Can you work these out from the drawing? Everything is in mm from the part's minimum corner. A direction names the side the tool comes from. Round coordinates to 2 decimals unless told otherwise and drop trailing zeros. Order: outer loops, then holes, each group sorted by start corner. A loop starts at its lowest first (then second) coordinate and runs counter-clockwise, first axis right, second up. Notation, with made-up numbers: (49, -14.75) -> (78, -14.75) arc R23 ccw to (78, 1.25) -> close; hole circle Ø4 at (-34.75, -30). An arc over 180 degrees is marked (long way). One line per item, written item: value.
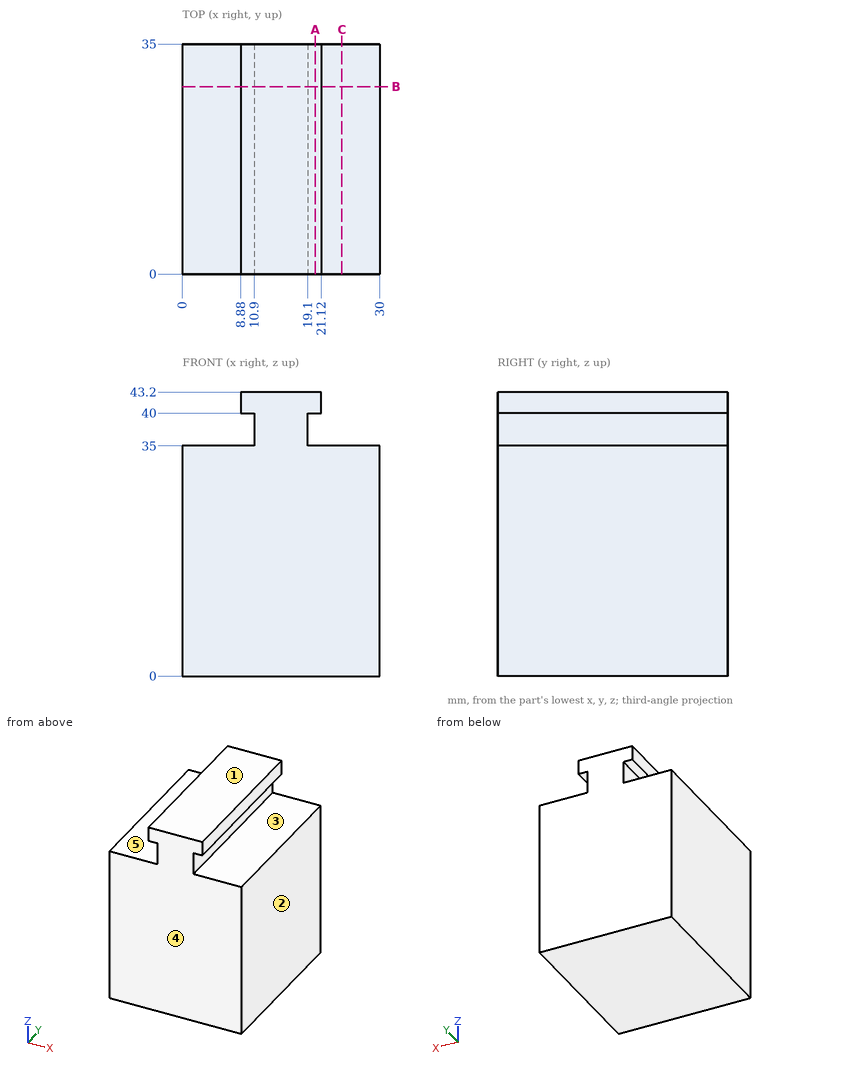
Q1. Which directions (+Z, -Z, +X, -X, +Y, -Y) give clear straight access to the entire face, cutting with the end or side of a thin tool? Please do the marked faces 4 and 5.
Answers:
face 4: +Z, -Z, +X, -X, -Y
face 5: -X, +Y, -Y
Q2. I want a section at C-C on x = 24.25. Write out the boundary of the cut face in (y, z), then the cut area to 4 significant figures.
Answers:
outline: (0, 0) -> (35, 0) -> (35, 35) -> (0, 35) -> close
area: 1,225 mm2
Q3. For P1, Ø2.5, axis at y = 22, z = 38, coming from the +X side; P2, Ø5.5, axis at y = 18, z = 38.5, coming from the -X side; P3, Ø1, axis at x = 22.5, y = 9, coming from the +Z side, each with a flat end and sliding along its axis, tell me the tip position at first contact or that it passes through.
Answers:
P1: x = 19.1
P2: x = 8.88
P3: z = 35
Q4. I want a section at B-B on y = 28.5. Write out the boundary of the cut face in (x, z).
Answers:
outline: (0, 0) -> (30, 0) -> (30, 35) -> (19.1, 35) -> (19.1, 40) -> (21.12, 40) -> (21.12, 43.2) -> (8.88, 43.2) -> (8.88, 40) -> (10.9, 40) -> (10.9, 35) -> (0, 35) -> close
Q5. If we mould it in two halves opening along Z, with no side actions, what happens to the marked faces 1, 2 and 3? For each: pulls with the +Z half, pulls with the -Z half, needs draft (parallel to the pull), parting line crosses it, or undercut.
Answers:
face 1: pulls with the +Z half
face 2: needs draft
face 3: undercut
Q6. I need wall thicknesses on line 1 along Z through (x, y) = (3, 16.5); line 2 along X through (y, z) = (7.5, 41.5); line 3 along X through (y, z) = (28, 37.5). Which ranges of each line are inside material? Lowest first, please.
Answers:
line 1: 0 to 35
line 2: 8.88 to 21.12
line 3: 10.9 to 19.1
Q7. I want a section at A-A on x = 20.25. Write out the boundary of the cut face in (y, z), then the cut area to 3 significant figures.
Answers:
outline: (0, 0) -> (35, 0) -> (35, 35) -> (0, 35) -> close; (0, 40) -> (35, 40) -> (35, 43.2) -> (0, 43.2) -> close
area: 1,340 mm2
